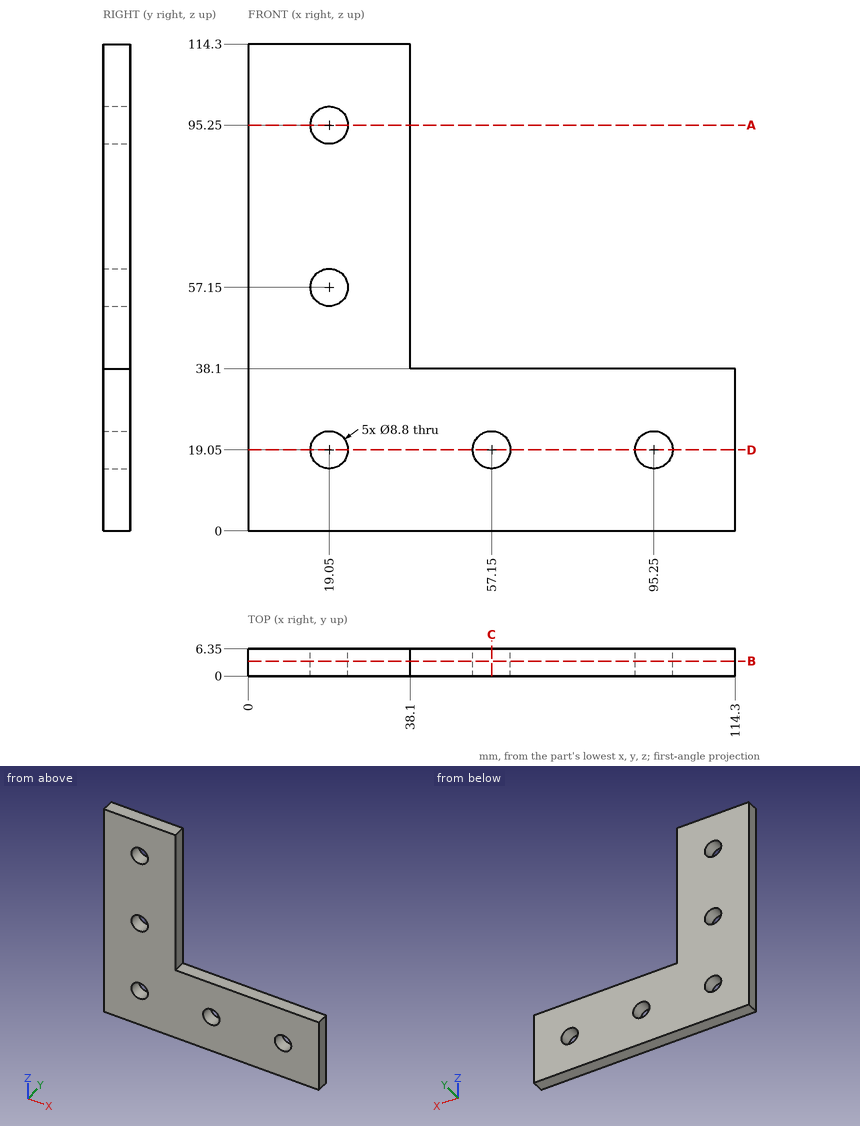
Answer from the drawing. Dimensions are ordinates in mm from the lowest x, y and z of the part. Round coordinates to 2 decimals unless told otherwise and drop trailing zeros. Loops run counter-clockwise (first coordinate to the right, second up) from the corner with the lowest first, then second, coordinate; pieces in that order, holes last.
Q1. Section C-C on x = 57.15 is taken. Write down the section's boundary in (y, z).
Q2. Each of these flat-tipped pins is pushed along its axis until it touches: pin 1 (1.9 mm diameter, centred on x = 60, y = 3, fed in from +Z); pin 2 (2 mm diameter, centred on x = 95.5, z = 40.5, fed in from +Y). Where does it stop, or does it pass through?
Q3. Consider probe 1 along Z at (x, y) = (19.05, 5); probe 2 along Z at (x, y) = (95.25, 2.25); probe 3 along X at (y, z) = (2.25, 51.5). Determine where each line is inside the solid, lowest interval first.
Q4. Section A-A on z = 95.25 is taken. Write down the section's boundary in (x, y).
Q5. Section D-D on z = 19.05 is taken. Write down the section's boundary in (x, y), and give its area (3 significant figures).
Q6. Section B-B on y = 3.5 is taken. Write down the section's boundary in (x, z), and give its area (3 significant figures).
Output:
1. outline: (0, 0) - (6.35, 0) - (6.35, 14.65) - (0, 14.65) - close; (0, 23.45) - (6.35, 23.45) - (6.35, 38.1) - (0, 38.1) - close
2. pin 1: stops at z = 38.1
2. pin 2: passes through
3. probe 1: z = 0 to 14.65, 23.45 to 52.75, 61.55 to 90.85, 99.65 to 114.3
3. probe 2: z = 0 to 14.65, 23.45 to 38.1
3. probe 3: x = 0 to 38.1
4. outline: (0, 0) - (14.65, 0) - (14.65, 6.35) - (0, 6.35) - close; (23.45, 0) - (38.1, 0) - (38.1, 6.35) - (23.45, 6.35) - close
5. outline: (0, 0) - (14.65, 0) - (14.65, 6.35) - (0, 6.35) - close; (23.45, 0) - (52.75, 0) - (52.75, 6.35) - (23.45, 6.35) - close; (61.55, 0) - (90.85, 0) - (90.85, 6.35) - (61.55, 6.35) - close; (99.65, 0) - (114.3, 0) - (114.3, 6.35) - (99.65, 6.35) - close
5. area: 558 mm2
6. outline: (0, 0) - (114.3, 0) - (114.3, 38.1) - (38.1, 38.1) - (38.1, 114.3) - (0, 114.3) - close; hole circle Ø8.8 at (19.05, 19.05); hole circle Ø8.8 at (19.05, 57.15); hole circle Ø8.8 at (19.05, 95.25); hole circle Ø8.8 at (57.15, 19.05); hole circle Ø8.8 at (95.25, 19.05)
6. area: 6,950 mm2
